Check sheet for the modelled part. Datum: model origin and axes. Units: mm. Give positions to 0.01 mm unless a question says otherwise; leave off trailing zeros. Order: outer loops, then holes, each group sorted by start corner. A loop starts at its lowest first (then second) coordinate and runs counter-clockwise, first axis right, second up. Notation, with made-up numbers: (-3, -32) - (22, -32) arc R31 ccw to (22, -5) - close; hole circle Ø3 at (49.25, 25.25). An arc over 180 degrees is marked (long way). Answer in a Markdown table with one row per item.
from build123d import *

# Parameters (mm, degrees)
F1_DEPTH = 6.35
F2_DEPTH = 12.7
F3_DEPTH = 24.638


with BuildPart() as f1:
    # F0 (on Front) → F1 (new body)
    with BuildSketch(Plane.XZ):
        with BuildLine():
            Line((-1.0786289811, 247.65), (-10.6036289811, 247.65))
            Line((-10.6036289811, 247.65), (-10.6036289811, -38.1))
            Line((-10.6036289811, -38.1), (2.0963710189, -38.1))
            Line((2.0963710189, -38.1), (14.7963710189, -38.1))
            Line((14.7963710189, -38.1), (14.7963710189, 247.65))
            Line((14.7963710189, 247.65), (5.2713710189, 247.65))
            ThreePointArc((5.2713710189, 247.65), (2.0963710189, 244.475), (-1.0786289811, 247.65))
        make_face()
        with BuildLine():
            ThreePointArc((8.4463710189, -25.4), (6.5864990794, -29.8901280605), (2.0963710189, -31.75))
            ThreePointArc((2.0963710189, -31.75), (-2.3937570416, -20.9098719395), (8.4463710189, -25.4))
        make_face(mode=Mode.SUBTRACT)
        with BuildLine():
            Line((-1.0786289811, 260.35), (-10.6036289811, 260.35))
            Line((-10.6036289811, 260.35), (-10.6036289811, 247.65))
            Line((-10.6036289811, 247.65), (-1.0786289811, 247.65))
            ThreePointArc((-1.0786289811, 247.65), (-0.1486930114, 249.8950640303), (2.0963710189, 250.825))
            Line((2.0963710189, 250.825), (2.0963710189, 257.175))
            ThreePointArc((2.0963710189, 257.175), (-0.1486930114, 258.1049359697), (-1.0786289811, 260.35))
        make_face()
        with BuildLine():
            Line((14.7963710189, 247.65), (14.7963710189, 260.35))
            Line((14.7963710189, 260.35), (5.2713710189, 260.35))
            ThreePointArc((5.2713710189, 260.35), (4.3414350492, 258.1049359697), (2.0963710189, 257.175))
            Line((2.0963710189, 257.175), (2.0963710189, 250.825))
            ThreePointArc((2.0963710189, 250.825), (4.3414350492, 249.8950640303), (5.2713710189, 247.65))
            Line((5.2713710189, 247.65), (14.7963710189, 247.65))
        make_face()
        with BuildLine():
            ThreePointArc((8.4463710189, -25.4), (-2.3937570416, -20.9098719395), (2.0963710189, -31.75))
            ThreePointArc((2.0963710189, -31.75), (6.5864990794, -29.8901280605), (8.4463710189, -25.4))
        make_face()
        with BuildLine():
            Line((2.0963710189, 266.7), (-10.6036289811, 266.7))
            Line((-10.6036289811, 266.7), (-10.6036289811, 260.35))
            Line((-10.6036289811, 260.35), (-1.0786289811, 260.35))
            ThreePointArc((-1.0786289811, 260.35), (-0.1486930114, 262.5950640303), (2.0963710189, 263.525))
            Line((2.0963710189, 263.525), (2.0963710189, 266.7))
        make_face()
        with BuildLine():
            Line((14.7963710189, 266.7), (2.0963710189, 266.7))
            Line((2.0963710189, 266.7), (2.0963710189, 263.525))
            ThreePointArc((2.0963710189, 263.525), (4.3414350492, 262.5950640303), (5.2713710189, 260.35))
            Line((5.2713710189, 260.35), (14.7963710189, 260.35))
            Line((14.7963710189, 260.35), (14.7963710189, 266.7))
        make_face()
        with BuildLine():
            Line((2.0963710189, 247.65), (-1.0786289811, 247.65))
            ThreePointArc((-1.0786289811, 247.65), (2.0963710189, 244.475), (5.2713710189, 247.65))
            Line((5.2713710189, 247.65), (2.0963710189, 247.65))
        make_face()
        with BuildLine():
            Line((5.2713710189, 260.35), (2.0963710189, 260.35))
            Line((2.0963710189, 260.35), (2.0963710189, 257.175))
            ThreePointArc((2.0963710189, 257.175), (4.3414350492, 258.1049359697), (5.2713710189, 260.35))
        make_face()
        with BuildLine():
            ThreePointArc((2.0963710189, 250.825), (-0.1486930114, 249.8950640303), (-1.0786289811, 247.65))
            Line((-1.0786289811, 247.65), (2.0963710189, 247.65))
            Line((2.0963710189, 247.65), (2.0963710189, 250.825))
        make_face()
        with BuildLine():
            Line((2.0963710189, 260.35), (2.0963710189, 263.525))
            ThreePointArc((2.0963710189, 263.525), (-0.1486930114, 262.5950640303), (-1.0786289811, 260.35))
            Line((-1.0786289811, 260.35), (2.0963710189, 260.35))
        make_face()
        with BuildLine():
            Line((2.0963710189, 260.35), (-1.0786289811, 260.35))
            ThreePointArc((-1.0786289811, 260.35), (-0.1486930114, 258.1049359697), (2.0963710189, 257.175))
            Line((2.0963710189, 257.175), (2.0963710189, 260.35))
        make_face()
        with BuildLine():
            ThreePointArc((5.2713710189, 260.35), (4.3414350492, 262.5950640303), (2.0963710189, 263.525))
            Line((2.0963710189, 263.525), (2.0963710189, 260.35))
            Line((2.0963710189, 260.35), (5.2713710189, 260.35))
        make_face()
        with BuildLine():
            Line((2.0963710189, 250.825), (2.0963710189, 247.65))
            Line((2.0963710189, 247.65), (5.2713710189, 247.65))
            ThreePointArc((5.2713710189, 247.65), (4.3414350492, 249.8950640303), (2.0963710189, 250.825))
        make_face()
    extrude(amount=F1_DEPTH)

    # F0 (on Front) → F2 (join)
    with BuildSketch(Plane.XZ):
        with BuildLine():
            ThreePointArc((8.4463710189, -25.4), (-2.3937570416, -20.9098719395), (2.0963710189, -31.75))
            ThreePointArc((2.0963710189, -31.75), (6.5864990794, -29.8901280605), (8.4463710189, -25.4))
        make_face()
    extrude(amount=F2_DEPTH)

    # F0 (on Front) → F3 (cut)
    with BuildSketch(Plane.XZ):
        with BuildLine():
            Line((2.0963710189, 250.825), (2.0963710189, 247.65))
            Line((2.0963710189, 247.65), (5.2713710189, 247.65))
            ThreePointArc((5.2713710189, 247.65), (4.3414350492, 249.8950640303), (2.0963710189, 250.825))
        make_face()
        with BuildLine():
            ThreePointArc((2.0963710189, 250.825), (-0.1486930114, 249.8950640303), (-1.0786289811, 247.65))
            Line((-1.0786289811, 247.65), (2.0963710189, 247.65))
            Line((2.0963710189, 247.65), (2.0963710189, 250.825))
        make_face()
        with BuildLine():
            Line((2.0963710189, 247.65), (-1.0786289811, 247.65))
            ThreePointArc((-1.0786289811, 247.65), (2.0963710189, 244.475), (5.2713710189, 247.65))
            Line((5.2713710189, 247.65), (2.0963710189, 247.65))
        make_face()
        with BuildLine():
            ThreePointArc((5.2713710189, 260.35), (4.3414350492, 262.5950640303), (2.0963710189, 263.525))
            Line((2.0963710189, 263.525), (2.0963710189, 260.35))
            Line((2.0963710189, 260.35), (5.2713710189, 260.35))
        make_face()
        with BuildLine():
            Line((2.0963710189, 260.35), (2.0963710189, 263.525))
            ThreePointArc((2.0963710189, 263.525), (-0.1486930114, 262.5950640303), (-1.0786289811, 260.35))
            Line((-1.0786289811, 260.35), (2.0963710189, 260.35))
        make_face()
        with BuildLine():
            Line((2.0963710189, 260.35), (-1.0786289811, 260.35))
            ThreePointArc((-1.0786289811, 260.35), (-0.1486930114, 258.1049359697), (2.0963710189, 257.175))
            Line((2.0963710189, 257.175), (2.0963710189, 260.35))
        make_face()
        with BuildLine():
            Line((5.2713710189, 260.35), (2.0963710189, 260.35))
            Line((2.0963710189, 260.35), (2.0963710189, 257.175))
            ThreePointArc((2.0963710189, 257.175), (4.3414350492, 258.1049359697), (5.2713710189, 260.35))
        make_face()
    extrude(amount=F3_DEPTH, mode=Mode.SUBTRACT)


solid = f1.part
(1) Gauge pin test, flat ends, axial feed: P1, Ø4, axis at x = 3.5, z = 94.5, coming from the -Y side; P2, Ø4, axis at y = -7, z = 42.5, coming from the +X side; P3, Ø1.5, axis at x = 0, y = -8, coming from the +Z side. Record the tip position at first contact, or that the pin passes through.
Geometry says:
| item | result |
|---|---|
| P1 | y = -6.35 |
| P2 | x = 14.8 |
| P3 | z = -19.19 |
(2) Cross-section at A-A, the plane z = 226.5. Record the cut outline in (x, y), then the cut area to 3 significant figures.
Geometry says:
| item | result |
|---|---|
| outline | (-10.6, -6.35) - (14.8, -6.35) - (14.8, 0) - (-10.6, 0) - close |
| area | 161 mm² |
(3) Thickness scan on L1, parallel to Y at x = 6, z = 86; L2, parallel to Z at x = 2, y = -10. Record the ranges inside material, lowest first.
Geometry says:
| item | result |
|---|---|
| L1 | -6.35 to 0 |
| L2 | -31.75 to -19.05 |
